Autodesk Inventor part; units mm, degrees
ref_plane "Querschnittsebene" through (113.874605, 5.547406, 0) normal (-0.995868, -0.090813, 0) x (0, 0, 1)
ref_plane "Arbeitsebene2" through (114.380472, 0, 0) normal (-1, 0, 0) x (0, 0, 1)
ref_plane "Arbeitsebene3" through (-9.997237, 0.815845, 0) normal (0.99382, -0.1110038, 0) x (0, 0, 1)
sketch "Skizzenpfad" plane through (0, 0, 0) normal (0, 0, 1) x (1, 0, 0)
  arc A0 (114.343934, -5.570303) -> (113.874605, 5.547406) centre (114.380472, 0) ccw
  arc A1 (-8.729894, 6.240184) -> (-10.033775, -4.754459) centre (-9.997237, 0.815845) ccw
  arc A2 (24.703327, -1.571154) -> (24.994596, -1.605239) centre (24.999094, -0.305247) ccw
  arc A3 (34.994536, -1.639838) -> (35.117091, -1.634474) centre (34.999034, -0.339846) ccw
  line L0 (35.117091, -1.634474) -> (113.874605, 5.547406)
  line L1 (114.343934, -5.570303) -> (-10.033775, -4.754459)
  line L2 (-8.729894, 6.240184) -> (24.703327, -1.571154)
  line L3 (24.994596, -1.605239) -> (34.994536, -1.639838)
ref_plane "Querschnittsebene" through (113.874605, 5.547406, 0) normal (-0.995868, -0.090813, 0) x (0, 0, 1)
ref_plane "Arbeitsebene2" through (114.380472, 0, 0) normal (-1, 0, 0) x (0, 0, 1)
ref_plane "Arbeitsebene3" through (-9.997237, 0.815845, 0) normal (0.99382, -0.1110038, 0) x (0, 0, 1)
sketch "Querschnitt" plane through (113.874605, 5.547406, 0) normal (-0.995868, -0.090813, 0) x (0, 0, 1)
  line L0 (-3, 0.3) -> (3, 0.3)
  line L1 (3, 0.3) -> (3, -0.3)
  line L2 (3, -0.3) -> (-3, -0.3)
  line L3 (-3, -0.3) -> (-3, 0.3)
  line L4 (-3, 0) -> (3, 0) construction
  point P0 (0, 0)
  point P1 (0, 0)
  dimension "d0" = 6
  dimension "d4" = 0.3
  dimension "d5" = 0.3
sweep "Riemen" add profiles "Querschnitt" path "Skizzenpfad"
equation "\"d0\" = da_B"
equation "\"d4\" = da_a"
equation "\"d5\" = da_a2"
equation "\"da_B\" = 6"
equation "\"da_pb\" = 2.5"
equation "\"da_L\" = 285"
equation "\"da_a\" = 0.3"
equation "\"da_S\" = 1.5"
equation "\"da_Beta\" = 20deg"
equation "\"da_Ht\" = 0.7"
equation "\"da_H\" = 1.3"
equation "\"da_a2\" = 0.3"
properties part number "Zahnriemen" material "Rubber"
For this review, take the finished solid that the model builds, in its own axes (mm). A direction names the side the tool comes from. Round coordinates to 2 decimals unless told otherwise and drop trailing zeros. Write each loop counter-clockwise with the first axis right and the second up, starting at its lowest first coordinate (ties: lowest second). Pieces come first, ordered by that corner, then holes. Notation, with made-up numbers: (86, -26) -> (122, -26) arc R12 cw to (122, -6) -> close; hole circle Ø10 at (-26, 64.5). An arc over 180 degrees is marked (long way). Put each result on its own line as item: value.
Q1. Consider section A-A on z = -1.8. State the section outline as (x, y) points.
Determined:
outline: (-10.04, -5.05) -> (114.34, -5.87) arc R5.87 ccw (long way) to (113.85, 5.85) -> (35.09, -1.34) arc R1 cw to (35, -1.34) -> (25, -1.31) arc R1 cw to (24.77, -1.28) -> (-8.66, 6.53) arc R5.87 ccw (long way) to start; hole (-10.03, -4.45) -> (114.35, -5.27) arc R5.27 ccw (long way) to (113.9, 5.25) -> (35.14, -1.93) arc R1.6 cw to (34.99, -1.94) -> (24.99, -1.91) arc R1.6 cw to (24.64, -1.86) -> (-8.8, 5.95) arc R5.27 ccw (long way) to start
Q2. The part is to be moulded in two halves that separate along Y. For faces 4 (the cylindrical face through (-15.84, 1.37, -0.04)), 5 (the flat face through (7.68, 2.1, -0.04)), 6 (the flat face through (67.3, 1.45, -3)), say which applies: released by +Y, released by -Y, zero draft, split by the parting line, or undercut.
Determined:
face 4: split by the parting line
face 5: undercut
face 6: zero draft
Q3. Machinability: for faces 1 (the flat face through (73.917, 2.205, 0.042)), 2 (the cylindrical face through (119.65, 0.1, 0.04)), 3 (the flat face through (53, 0, 3)), which of the approach directions +Z, -Z, +X, -X, +Y, -Y give a long, thin tool a straight path to every point of the face, cutting with its end or side? Answer none if there is none.
Determined:
face 1: +Z, -Z, +Y
face 2: +Z, -Z
face 3: +Z, +X, -X, +Y, -Y
Q4. To check wall thickness, follow L1, parallel to X at y = -2.25, z = -2.05; L2, parallel to Y at x = 2, z = 2.7; L3, parallel to Y at x = 55, z = -1. State the ranges of each line that lie inside material, in increasing order. Write a range as [from, to].
Determined:
L1: x = [-15, -14.28], [119.15, 119.8]
L2: y = [-5.13, -4.53], [3.43, 4.04]
L3: y = [-5.48, -4.88], [-0.12, 0.48]
Q5. Consider section B-B on y = 2.5. State the section outline as (x, z) points.
Determined:
outline: (-15.62, -3) -> (-14.99, -3) -> (-14.99, 3) -> (-15.62, 3) -> close; (5.96, -3) -> (8.6, -3) -> (8.6, 3) -> (5.96, 3) -> close; (77.15, -3) -> (83.76, -3) -> (83.76, 3) -> (77.15, 3) -> close; (119.02, -3) -> (119.69, -3) -> (119.69, 3) -> (119.02, 3) -> close
Q6. Consider section C-C on x = 41. State the section outline as (y, z) points.
Determined:
outline: (-5.39, -3) -> (-4.79, -3) -> (-4.79, 3) -> (-5.39, 3) -> close; (-1.4, -3) -> (-0.8, -3) -> (-0.8, 3) -> (-1.4, 3) -> close
Q7. Clearance check with flat-ended pins moving along their axes: pin 1 Ø2 at (x, z) = (102.5, -0.5) entering from +Y; pin 2 Ø1 at (x, z) = (83.5, -0.5) entering from -Y; pin 3 Ø3 at (x, y) = (15, 4) entering from +Z; pin 4 Ø1 at (x, z) = (29.5, -2) entering from -Y. State where each tip first meets the part, or that it passes through.
Determined:
pin 1: stops at y = 4.9
pin 2: stops at y = -5.67
pin 3: passes through
pin 4: stops at y = -5.32
